Could you check a few things on this drawing? It's one solid part, dimensions in mm from its lowest x, y, z. A direction names the side the tool comes from. Give positions to 0.01 mm unless a question says otherwise; leave off trailing zeros. Order: outer loops, then holes, each group sorted by start corner. A loop starts at its lowest first (then second) coordinate and runs counter-clockwise, first axis right, second up. Notation, with made-up numbers: (5, -30) -> (11, -30) arc R16 ccw to (11, -7) -> close; hole circle Ø10 at (25, 7.5). An arc over 180 degrees is marked (long way). Answer as a JSON object with one key per item and string values.
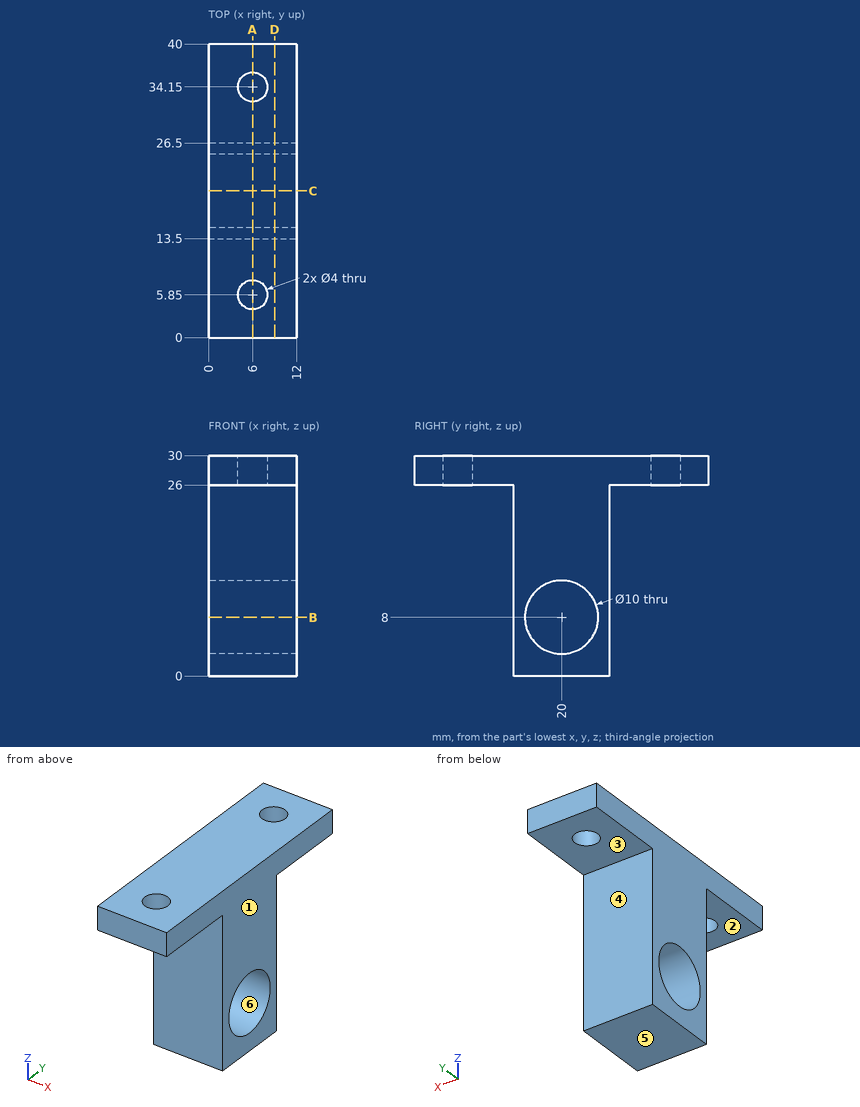
1. Please list where these lines run through material, in increasing order: L1, parallel to Y at x = 6, z = 28.9; L2, parallel to Y at x = 6.5, z = 2.5; L3, parallel to Y at x = 4, z = 8.25.
Worked answers:
{"L1": "0 to 3.85, 7.85 to 32.15, 36.15 to 40", "L2": "13.5 to 26.5", "L3": "13.5 to 15.01, 24.99 to 26.5"}
2. If we mould it in two halves opening along Z, with no side actions, what happens to the marked faces 4, 5 and 6? For each: +Z half, -Z half, draft (parallel to the pull), parting line (faces both ways), or undercut.
Worked answers:
{"face 4": "draft", "face 5": "-Z half", "face 6": "undercut"}
3. If we section it at A-A on x = 6: Please give me the cut outline in (y, z).
Worked answers:
{"outline": "(0, 26) -> (3.85, 26) -> (3.85, 30) -> (0, 30) -> close; (7.85, 26) -> (13.5, 26) -> (13.5, 0) -> (26.5, 0) -> (26.5, 26) -> (32.15, 26) -> (32.15, 30) -> (7.85, 30) -> close; (36.15, 26) -> (40, 26) -> (40, 30) -> (36.15, 30) -> close; hole circle Ø10 at (20, 8)"}
4. If we section it at B-B on z = 8: Please give me the cut outline in (x, y).
Worked answers:
{"outline": "(0, 13.5) -> (12, 13.5) -> (12, 15) -> (0, 15) -> close; (0, 25) -> (12, 25) -> (12, 26.5) -> (0, 26.5) -> close"}
5. Will these pins go through, and if not, where does the flat tip stop? pin 1 Ø3.5 at (x, y) = (7, 5.5) entering from -Z; pin 2 Ø5 at (y, z) = (15.5, 22.5) entering from -X; pin 3 Ø3.5 at (x, z) = (3.5, 8.5) entering from -Y; pin 4 Ø6 at (x, z) = (5.5, 14) entering from +Y.
Worked answers:
{"pin 1": "z = 26", "pin 2": "x = 0", "pin 3": "y = 13.5", "pin 4": "y = 26.5"}
6. If we section it at D-D on x = 9: Please give me the cut outline in (y, z).
Worked answers:
{"outline": "(0, 26) -> (13.5, 26) -> (13.5, 0) -> (26.5, 0) -> (26.5, 26) -> (40, 26) -> (40, 30) -> (0, 30) -> close; hole circle Ø10 at (20, 8)"}
7. For the marked faces 1, 2 and 3, which set-ups out of +Z, -Z, +X, -X, +Y, -Y let a thin tool reach every point of the face, with its end or its side?
Worked answers:
{"face 1": "+Z, -Z, +X, +Y, -Y", "face 2": "-Z, +X, -X, -Y", "face 3": "-Z, +X, -X, +Y"}
8. If we section it at C-C on y = 20: Please give me the cut outline in (x, z).
Worked answers:
{"outline": "(0, 0) -> (12, 0) -> (12, 3) -> (0, 3) -> close; (0, 13) -> (12, 13) -> (12, 30) -> (0, 30) -> close"}
